```python
from build123d import *

# Parameters (mm, degrees)
SKETCH_1_R      = 7.075
EXTRUDE_1_DEPTH = 6.85
EXTRUDE_START   = -1
SKETCH_2_R      = 7.075
SKETCH_2_R_2    = 5.575
EXTRUDE_2_DEPTH = 1
CHAMFER_1_SIZE  = 1


with BuildPart() as part:
    # 草图1 → 凸台-拉伸1 (new body)
    with BuildSketch(Plane.XY):
        with BuildLine():
            ThreePointArc((2.588190451, 9.659258263), (-10, 0), (2.588190451, -9.659258263))
            Line((2.588190451, -9.659258263), (18.11075361, -5.5))
            Line((18.11075361, -5.5), (159.28924639, -5.5))
            Line((159.28924639, -5.5), (174.811809549, -9.659258263))
            ThreePointArc((174.811809549, -9.659258263), (187.4, 0), (174.811809549, 9.659258263))
            Line((174.811809549, 9.659258263), (159.28924639, 5.5))
            Line((159.28924639, 5.5), (18.11075361, 5.5))
            Line((18.11075361, 5.5), (2.588190451, 9.659258263))
        make_face()
        with Locations(Location((0, 0, 0), (0, 0, 180))):
            Circle(SKETCH_1_R, mode=Mode.SUBTRACT)
        with Locations(Location((177.4, 0, 0), (0, 0, 180))):
            Circle(SKETCH_1_R, mode=Mode.SUBTRACT)
    extrude(amount=EXTRUDE_1_DEPTH)

    # 草图2 → 凸台-拉伸2 (add)
    # profile 1 of 2: a face of its own
    with BuildSketch(Plane.XY.offset(6.85).offset(EXTRUDE_START)):
        with Locations(Location((0, 0, 0), (0, 0, 180))):
            Circle(SKETCH_2_R)
        Circle(SKETCH_2_R_2, mode=Mode.SUBTRACT)
    # profile 2 of 2: a face of its own
    with BuildSketch(Plane.XY.offset(6.85).offset(EXTRUDE_START)):
        with Locations(Location((177.4, 0, 0), (0, 0, 180))):
            Circle(SKETCH_2_R)
        with Locations((177.4, 0)):
            Circle(SKETCH_2_R_2, mode=Mode.SUBTRACT)
    extrude(amount=EXTRUDE_2_DEPTH)

    # 倒角1
    chamfer_1_edges = [part.edges().sort_by_distance(p)[0] for p in [
        (187.4, 0, 6.85),
        (88.7, -5.5, 0),
        (10.34947203, -7.579629131, 0),
        (-10, 0, 0),
        (10.34947203, 7.579629131, 0),
        (88.7, 5.5, 0),
        (167.05052797, 7.579629131, 0),
        (187.4, 0, 0),
        (167.05052797, -7.579629131, 0),
        (167.05052797, 7.579629131, 6.85),
        (88.7, 5.5, 6.85),
        (10.34947203, 7.579629131, 6.85),
        (-10, 0, 6.85),
        (10.34947203, -7.579629131, 6.85),
        (88.7, -5.5, 6.85),
        (167.05052797, -7.579629131, 6.85),
    ]]
    chamfer(chamfer_1_edges, length=CHAMFER_1_SIZE)


solid = part.part
```
Read the model definition and answer for the solid it produces. Units are mm, in the model's axes. A direction names the side the tool comes from. Give positions to 0.01 mm unless a question says otherwise; leave off trailing zeros. Order: outer loops, then holes, each group sorted by start corner. A loop starts at its lowest first (then second) coordinate and runs counter-clockwise, first axis right, second up.
(1) Given pin 1 (2 mm diameter, centred on y = 2, z = 1, fed in from +X); pin 2 (4 mm diameter, centred on x = 57.5, z = 4.5, fed in from +Y); pin 3 (1.5 mm diameter, centred on x = 137.5, y = 5.5, fed in from +Z), each flat-ended and moving along its own axis, determine where each tip first touches the part or whether it passes through.
(2) Find section B-B (x = 0). Give the vertices of the cut face in (y, z) (3 decimals).
(3) Find section A-A (z = 4.5). Give the vertices of the cut face in (x, y) (3 decimals), plus the area to 3 significant figures.
(4) For faces 5 (the cylindrical face through (170.652, -2.125, 2.884)), 6 (the flat face through (10.18, -7.12, 6.34)), 7 (the flat face through (90, 5.5, 3)), determine the directions among +Z, -Z, +X, -X, +Y, -Y from which every point of the face is accessible in a straight line to the end or side of a thin tool.
(5) Straight lines are drawn through the part: L1, parallel to X at y = -0.5, z = 2.5; L2, parallel to Y at x = 0, z = 4.1 (3 decimals); L3, parallel to X at y = 4.25, z = 4.5. For each, find the intervals that lie inside material, in ascending order.
(6) Find section C-C (x = 116). Give the vertices of the cut face in (y, z), plus the area to 4 significant figures.
(7) For a pull along Y with two mould halves and no side action, classify faces 1 (the conical face through (-9.171, 0.235, 6.676)), 2 (the flat face through (172, -2, 5.85)), 3 (the flat face through (167.2, 7.1, 0.5)), 4 (the flat face through (166.94, -7.55, 3.39)) as released by +Y, released by -Y, zero draft, split by the parting line, or undercut.
Result sheet:
1. pin 1: stops at x = 187.35
1. pin 2: stops at y = 5.5
1. pin 3: stops at z = 6.6
2. outline: (-10, 1) - (-9, 0) - (-7.075, 0) - (-7.075, 5.85) - (-5.575, 5.85) - (-5.575, 6.85) - (-9, 6.85) - (-10, 5.85) - close; (5.575, 5.85) - (7.075, 5.85) - (7.075, 0) - (9, 0) - (10, 1) - (10, 5.85) - (9, 6.85) - (5.575, 6.85) - close
3. outline: (2.588, -9.659) - (18.111, -5.5) - (159.289, -5.5) - (174.812, -9.659) arc R10 ccw (long way) to (174.812, 9.659) - (159.289, 5.5) - (18.111, 5.5) - (2.588, 9.659) arc R10 ccw (long way) to start; hole circle Ø14.15 at (0, 0); hole circle Ø14.15 at (177.4, 0)
3. area: 2,130 mm2
4. face 5: -Z
4. face 6: +Z, -Y
4. face 7: +Z, -Z, +Y
5. L1: x = -9.99 to -7.06, 7.06 to 170.34, 184.46 to 187.39
5. L2: y = -10 to -7.075, 7.075 to 10
5. L3: x = -9.05 to -5.66, 5.66 to 171.74, 183.06 to 186.45
6. outline: (-5.5, 1) - (-4.5, 0) - (4.5, 0) - (5.5, 1) - (5.5, 5.85) - (4.5, 6.85) - (-4.5, 6.85) - (-5.5, 5.85) - close
6. area: 73.35 mm2
7. face 1: split by the parting line
7. face 2: undercut
7. face 3: released by +Y
7. face 4: released by -Y
